```python
from build123d import *

# Parameters (mm, degrees)
F0_W     = 19.05
F0_H     = 44.45
F1_DEPTH = 5.08
F2_W     = 10
F2_H     = 5
F3_DEPTH = 25.4
F4_R     = 2.54
F6_D     = 3.3
F6_DEPTH = 12.7
F6_TIP   = 0.9914200214


with BuildPart() as f1:
    # F0 (on Top) → F1 (new body)
    with BuildSketch(Plane.XY):
        Rectangle(F0_W, F0_H)
    extrude(amount=F1_DEPTH)

    # F2 (on face) → F3 (cut)
    with BuildSketch(Plane.XY.offset(5.08)):
        with Locations((0, 24.725)):
            Rectangle(F2_W, F2_H)
        with Locations((0, 19.725)):
            Rectangle(F2_W, F2_H)
    extrude(amount=-F3_DEPTH, mode=Mode.SUBTRACT)

    # F4
    f4_edges = [f1.edges().sort_by_distance(p)[0] for p in [
        (-5, 17.225, 2.54),
        (5, 17.225, 2.54),
    ]]
    fillet(f4_edges, radius=F4_R)

    # F6
    with Locations(Plane.XY.offset(5.08)):
        with Locations((-5, -18.415), (5, -18.415)):
            Hole(F6_D / 2, depth=F6_DEPTH)
            with Locations((0, 0, -(F6_DEPTH + F6_TIP / 2))):  # 118° drill point
                Cone(0, F6_D / 2, F6_TIP, mode=Mode.SUBTRACT)


solid = f1.part
```
Build history of the part. All positions in model axes, mm. A direction names the side the tool comes from. Round coordinates to 2 decimals unless told otherwise and drop trailing zeros. Write each loop counter-clockwise with the first axis right and the second up, starting at its lowest first coordinate (ties: lowest second). Pieces come first, ordered by that corner, then holes. Notation, with made-up numbers: (-23, 75) - (-4, 75) arc R26 ccw to (-4, 98) - close; hole circle Ø4 at (37.5, 35). An arc over 180 degrees is marked (long way). Answer as CSV lines item,"result".
Q1. Cut at B-B (z = 1.4). Write the cut outline in (x, y) (3 decimals), and give its area (3 significant figures).
Report:
outline,"(-9.525, -22.225) - (9.525, -22.225) - (9.525, 22.225) - (5, 22.225) - (5, 19.765) arc R2.54 cw to (2.46, 17.225) - (-2.46, 17.225) arc R2.54 cw to (-5, 19.765) - (-5, 22.225) - (-9.525, 22.225) - close; hole circle Ø3.3 at (-5, -18.415); hole circle Ø3.3 at (5, -18.415)"
area,"782 mm^2"
Q2. Pull direction Y, two halves, no side cores. Call faces 1 (the cylindrical face through (-4.276, 17.989, 2.504)), 2 (the cylindrical face through (6.216, -17.3, 2.504)), 3 (the flat face through (0, -22.225, 3)): +Y half, -Y half, draft (parallel to the pull), parting line (faces both ways), or undercut.
Report:
face 1,"+Y half"
face 2,"undercut"
face 3,"-Y half"
Q3. Drop flat-ended pins along their axis: pin 1 (4.5 mm diameter, centred on x = 5, y = -18.415, fed in from +Z); pin 2 (2 mm diameter, centred on x = 1, z = 3, fed in from +Y) (3 decimals). Give the stop position or say it passes through.
Report:
pin 1,"stops at z = 5.08"
pin 2,"stops at y = 17.225"
Q4. Tool access for faces 4 (the flat face through (-7, 22.225, 3)), 5 (the cylindrical face through (4.236, 17.949, 2.504)): list every direction of +Z, -Z, +X, -X, +Y, -Y with a clear straight run to the whole face (end or side of a thin tool).
Report:
face 4,"+Z, -Z, +X, -X, +Y"
face 5,"+Z, -Z, +Y"
Q5. Drill centre lines: probe 1 along Y at (x, z) = (2.25, 0.4) (3 decimals); probe 2 along Y at (x, z) = (-3.75, 2.8) (3 decimals); probe 3 along Y at (x, z) = (-6, 3.7) (3 decimals). Where is each one in solid material? Low to high. Write a range as [from, to].
Report:
probe 1,"y = [-22.225, 17.225]"
probe 2,"y = [-22.225, -19.492], [-17.338, 17.577]"
probe 3,"y = [-22.225, -19.727], [-17.103, 22.225]"
Q6. Cut at C-C (y = -18). Write the cut outline in (x, z) (3 decimals).
Report:
outline,"(-9.525, 0) - (-6.597, 0) - (-6.597, 5.08) - (-9.525, 5.08) - close; (-3.403, 0) - (3.403, 0) - (3.403, 5.08) - (-3.403, 5.08) - close; (6.597, 0) - (9.525, 0) - (9.525, 5.08) - (6.597, 5.08) - close"
Q7. Cut at A-A (x = -5.75). Write the cut outline in (y, z) (3 decimals), and give its area (3 significant figures).
Report:
outline,"(-22.225, 0) - (-19.885, 0) - (-19.885, 5.08) - (-22.225, 5.08) - close; (-16.945, 0) - (22.225, 0) - (22.225, 5.08) - (-16.945, 5.08) - close"
area,"211 mm^2"
